from build123d import *

# Parameters (mm, degrees)
SKETCH1_R           = 10.65
SKETCH1_R_2         = 8.65
BOSS_EXTRUDE1_DEPTH = 237
SKETCH2_R           = 3.5
CUT_EXTRUDE1_DEPTH  = 238.478093727
LPATTERN1_COUNT     = 2
LPATTERN1_PITCH     = 150
SKETCH3_W           = 1
SKETCH3_H           = 7


with BuildPart() as part:
    # Sketch1 → Boss-Extrude1 (new body)
    with BuildSketch(Plane.XY):
        Circle(SKETCH1_R)
        Circle(SKETCH1_R_2, mode=Mode.SUBTRACT)
    extrude(amount=BOSS_EXTRUDE1_DEPTH)

    # Sketch2 → Cut-Extrude1 (cut, symmetric)
    with BuildSketch(Plane(origin=(0, 0, 0), x_dir=(1, 0, 0), z_dir=(0, 1, 0))):
        with Locations(Location((0, -177, 0), (0, 0, 270))):
            Circle(SKETCH2_R)
    cut_extrude1 = extrude(amount=CUT_EXTRUDE1_DEPTH, both=True, mode=Mode.SUBTRACT)

    # LPattern1: Cut-Extrude1 ×2
    with Locations(*[(0, 0, -i * LPATTERN1_PITCH) for i in range(1, LPATTERN1_COUNT)]):
        add(cut_extrude1, mode=Mode.SUBTRACT)

    # Sketch3 → Cut-Revolve1 (revolve, cut)
    with BuildSketch(Plane(origin=(0, 0, 0), x_dir=(1, 0, 0), z_dir=(0, 1, 0)), mode=Mode.PRIVATE) as cut_revolve1_sk:
        with Locations((-10.15, -233.5)):
            Rectangle(SKETCH3_W, SKETCH3_H)
    revolve(cut_revolve1_sk.sketch.rotate(Axis((0, 0, 237), (0, 0, -1)), 180), axis=Axis((0, 0, 237), (0, 0, -1)), mode=Mode.SUBTRACT)


solid = part.part
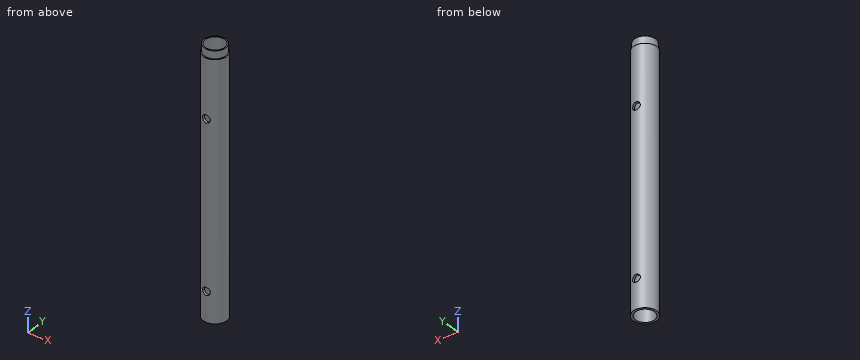
Check sheet for the modelled part. Datum: model origin and axes. Units: mm. Give positions to 0.01 mm unless a question says otherwise; leave off trailing zeros. Write each loop counter-clockwise with the first axis right and the second up, starting at its lowest first coordinate (ties: lowest second). Pieces come first, ordered by that corner, then holes. Notation, with made-up numbers: (2.25, -14.75) -> (23.25, -14.75) arc R21 cw to (23.25, -10.75) -> close; hole circle Ø11 at (20, -28.5). An arc over 180 degrees is marked (long way). Use one line per item in the form item = value. Start each with the question number.
1. Section check A-A (x = 0). Record the cut outline in (y, z), and give its area (3 significant figures).
2. Section check D-D (z = 27). Record the cut outline in (x, y), and give its area (3 significant figures).
3. Section check B-B (y = -4). Record the cut outline in (x, z), and give its area (3 significant figures).
4. Go/stop test with flat-tipped pins: P1, Ø4, axis at x = 0, z = 177, coming from the +Y side; P2, Ø1.5, axis at y = -1.5, z = 172, coming from the -X side; P3, Ø12, axis at x = -7.5, z = 82.5, coming from the -Y side; P4, Ø5, axis at x = -5, z = 62, coming from the -Y side. Record where each tip stops, or that it passes through.
5. Section check C-C (z = 211.5). Record the cut outline in (x, y).
6. Thickness scan on line 1 along Z through (x, y) = (0, -9.85); line 2 along Z through (x, y) = (0, 9.1); line 3 along Y through (x, z) = (0, 38). Record the ranges inside material, lowest first. Write a range as from..to.
Conclusion:
q1.outline = (-10.65, 0) -> (-8.65, 0) -> (-8.65, 23.5) -> (-10.65, 23.5) -> close; (-10.65, 30.5) -> (-8.65, 30.5) -> (-8.65, 173.5) -> (-10.65, 173.5) -> close; (-10.65, 180.5) -> (-8.65, 180.5) -> (-8.65, 237) -> (-9.65, 237) -> (-9.65, 230) -> (-10.65, 230) -> close; (8.65, 0) -> (10.65, 0) -> (10.65, 23.5) -> (8.65, 23.5) -> close; (8.65, 30.5) -> (10.65, 30.5) -> (10.65, 173.5) -> (8.65, 173.5) -> close; (8.65, 180.5) -> (10.65, 180.5) -> (10.65, 230) -> (9.65, 230) -> (9.65, 237) -> (8.65, 237) -> close
q1.area = 878 mm²
q2.outline = (-3.5, -10.06) -> (-3.5, -7.91) arc R8.65 cw to (-3.5, 7.91) -> (-3.5, 10.06) arc R10.65 ccw to start; (3.5, -10.06) arc R10.65 ccw to (3.5, 10.06) -> (3.5, 7.91) arc R8.65 cw to (3.5, -7.91) -> close
q2.area = 92.6 mm²
q3.outline = (-9.87, 0) -> (-7.67, 0) -> (-7.67, 237) -> (-8.78, 237) -> (-8.78, 230) -> (-9.87, 230) -> close; (7.67, 0) -> (9.87, 0) -> (9.87, 230) -> (8.78, 230) -> (8.78, 237) -> (7.67, 237) -> close
q3.area = 1,030 mm²
q4.P1 = through
q4.P2 = -10.62
q4.P3 = -10.54
q4.P4 = -10.35
q5.outline = circle Ø21.3 at (0, 0); hole circle Ø17.3 at (0, 0)
q6.line_1 = 0..23.5, 30.5..173.5, 180.5..230
q6.line_2 = 0..23.5, 30.5..173.5, 180.5..237
q6.line_3 = -10.65..-8.65, 8.65..10.65
